from build123d import *

# Parameters (mm, degrees)
CROQUIS1_R              = 1.5
CROQUIS1_R_2            = 1.499997567
CROQUIS1_R_3            = 1.499999659
SALIENTE_EXTRUIR1_DEPTH = 2


with BuildPart() as part:
    # Croquis1 → Saliente-Extruir1 (new body)
    with BuildSketch(Plane.XY):
        with BuildLine():
            Line((-41.931739537, 35.719555975), (-21.729231, 5.566101))
            ThreePointArc((-21.729231, 5.566101), (-20.036969421, 4.8e-08), (-21.729230683, -5.566101))
            Line((-21.729230683, -5.566101), (-41.931739683, -35.719556))
            ThreePointArc((-41.931739683, -35.719556), (-40.113877545, -46.255199079), (-29.502526011, -44.949972494))
            Line((-29.502526011, -44.949972494), (-23.17774412, -37.243793058))
            ThreePointArc((-23.17774412, -37.243793058), (-17.619189001, -31.253867186), (-11.353005357, -26.008708515))
            ThreePointArc((-11.353005357, -26.008708515), (-8.734615775, -24.660409187), (-5.826392082, -24.195532826))
            Line((-5.826392082, -24.195532826), (-8.2e-08, -24.195532826))
            Line((-8.2e-08, -24.195532826), (5.826391918, -24.195532937))
            ThreePointArc((5.826391918, -24.195532937), (8.734615571, -24.66040906), (11.3530052, -26.008708126))
            ThreePointArc((11.3530052, -26.008708126), (17.61928276, -31.253858591), (23.177925918, -37.243793826))
            Line((23.177925918, -37.243793826), (29.502525918, -44.949971826))
            ThreePointArc((29.502525918, -44.949971826), (40.113877545, -46.255199018), (41.931739905, -35.719555809))
            Line((41.931739905, -35.719555809), (40.742639905, -33.944752809))
            ThreePointArc((40.742639905, -33.944752809), (40.308182186, -27.575684066), (45.596686, -23.999999855))
            Line((45.596686, -23.999999855), (66.596686, -23.999999855))
            ThreePointArc((66.596686, -23.999999855), (68.20025333, -23.53546267), (69.307209533, -22.285714318))
            ThreePointArc((69.307209533, -22.285714318), (70.783151209, -20.619383034), (72.921241131, -20.000000062))
            Line((72.921241131, -20.000000062), (107.612588131, -20.000000062))
            ThreePointArc((107.612588131, -20.000000062), (110.006914278, -19.249811766), (111.54509388, -17.267494009))
            ThreePointArc((111.54509388, -17.267494009), (113.827321023, -8.772459026), (114.473968651, -5.93e-07))
            ThreePointArc((114.473968651, -5.93e-07), (113.827320947, 8.772458604), (111.545093444, 17.267494286))
            ThreePointArc((111.545093444, 17.267494286), (110.006913893, 19.249811756), (107.612588, 20))
            Line((107.612588, 20), (72.921241, 20))
            ThreePointArc((72.921241, 20), (70.783151239, 20.619383073), (69.307209698, 22.285714308))
            ThreePointArc((69.307209698, 22.285714308), (68.200253441, 23.535462771), (66.596686, 24))
            Line((66.596686, 24), (45.596686, 24))
            ThreePointArc((45.596686, 24), (40.308182457, 27.575684295), (40.74263977, 33.944752888))
            Line((40.74263977, 33.944752888), (41.93173977, 35.719555888))
            ThreePointArc((41.93173977, 35.719555888), (40.113879793, 46.255201891), (29.502526087, 44.949972367))
            Line((29.502526087, 44.949972367), (23.177744038, 37.243793232))
            ThreePointArc((23.177744038, 37.243793232), (17.619188919, 31.25386736), (11.353005274, 26.008708689))
            ThreePointArc((11.353005274, 26.008708689), (8.734615693, 24.660409361), (5.826392, 24.195533))
            Line((5.826392, 24.195533), (0, 24.195533))
            Line((0, 24.195533), (-5.826392, 24.195533111))
            ThreePointArc((-5.826392, 24.195533111), (-8.734615653, 24.660409234), (-11.353005282, 26.0087083))
            ThreePointArc((-11.353005282, 26.0087083), (-17.619282842, 31.253858765), (-23.177926, 37.243794))
            Line((-23.177926, 37.243794), (-29.502526, 44.949972))
            ThreePointArc((-29.502526, 44.949972), (-40.113877138, 46.255198613), (-41.931739537, 35.719555975))
        make_face()
        with Locations((59.75, -15.25)):
            Circle(CROQUIS1_R, mode=Mode.SUBTRACT)
        with Locations((-15.25, -15.25)):
            Circle(CROQUIS1_R, mode=Mode.SUBTRACT)
        with Locations((35.493242084, -40.033283689)):
            Circle(CROQUIS1_R, mode=Mode.SUBTRACT)
        with Locations((107.612588, -15.5)):
            Circle(CROQUIS1_R, mode=Mode.SUBTRACT)
        with Locations((-35.493241837, -40.033283897)):
            Circle(CROQUIS1_R, mode=Mode.SUBTRACT)
        with Locations((15.25, 15.25)):
            Circle(CROQUIS1_R, mode=Mode.SUBTRACT)
        with Locations((59.75, 15.25)):
            Circle(CROQUIS1_R, mode=Mode.SUBTRACT)
        with Locations((-25.371621, -27.641642)):
            Circle(CROQUIS1_R, mode=Mode.SUBTRACT)
        with Locations((-25.371621, 27.641642)):
            Circle(CROQUIS1_R, mode=Mode.SUBTRACT)
        with Locations((35.493244203, 40.033286852)):
            Circle(CROQUIS1_R_2, mode=Mode.SUBTRACT)
        with Locations((107.612588, 15.5)):
            Circle(CROQUIS1_R, mode=Mode.SUBTRACT)
        with Locations((-35.493241659, 40.033283492)):
            Circle(CROQUIS1_R_3, mode=Mode.SUBTRACT)
        with Locations((90.249999894, -15.249999839)):
            Circle(CROQUIS1_R, mode=Mode.SUBTRACT)
        with Locations((90.24999988, 15.250000209)):
            Circle(CROQUIS1_R, mode=Mode.SUBTRACT)
        with Locations((-15.25, 15.25)):
            Circle(CROQUIS1_R, mode=Mode.SUBTRACT)
        with Locations((25.371621, -27.641642)):
            Circle(CROQUIS1_R, mode=Mode.SUBTRACT)
        with Locations((15.25, -15.25)):
            Circle(CROQUIS1_R, mode=Mode.SUBTRACT)
        with Locations((25.371621, 27.641642)):
            Circle(CROQUIS1_R, mode=Mode.SUBTRACT)
        with BuildLine():
            Line((98.473924, 4.165983), (66.629579, 4.165983))
            ThreePointArc((66.629579, 4.165983), (63.80116944, 6.88617712), (66.409010926, 9.818500341))
            ThreePointArc((66.409010926, 9.818500341), (75.942438766, 10.701918647), (85.446477477, 11.859468837))
            ThreePointArc((85.446477477, 11.859468837), (86.461547798, 11.633214666), (87.383984261, 11.152933833))
            ThreePointArc((87.383984261, 11.152933833), (90.700963866, 10.270378747), (93.80542655, 11.734471854))
            ThreePointArc((93.80542655, 11.734471854), (96.321235225, 12.908534532), (98.995308731, 12.162178491))
            ThreePointArc((98.995308731, 12.162178491), (100.881174903, 9.908695061), (101.470839807, 7.02998457))
            ThreePointArc((101.470839807, 7.02998457), (100.546603986, 4.997112873), (98.473924, 4.165983))
        make_face(mode=Mode.SUBTRACT)
        with BuildLine():
            Line((66.596686, -22), (45.596686, -22))
            ThreePointArc((45.596686, -22), (44.596686, -21), (45.596686, -20))
            Line((45.596686, -20), (66.596686, -20))
            ThreePointArc((66.596686, -20), (67.596686, -21), (66.596686, -22))
        make_face(mode=Mode.SUBTRACT)
        with BuildLine():
            Line((66.596686, 22), (45.596686, 22))
            ThreePointArc((45.596686, 22), (44.596686, 21), (45.596686, 20))
            Line((45.596686, 20), (66.596686, 20))
            ThreePointArc((66.596686, 20), (67.596686, 21), (66.596686, 22))
        make_face(mode=Mode.SUBTRACT)
        with BuildLine():
            Line((98.473923843, -4.165983), (66.629579, -4.165983))
            ThreePointArc((66.629579, -4.165983), (63.801171492, -6.886177421), (66.409011186, -9.818500536))
            ThreePointArc((66.409011186, -9.818500536), (75.942439193, -10.70191878), (85.446478074, -11.859468919))
            ThreePointArc((85.446478074, -11.859468919), (86.461548299, -11.633214373), (87.383984575, -11.152933205))
            ThreePointArc((87.383984575, -11.152933205), (90.700964079, -10.270378355), (93.805426592, -11.734471456))
            ThreePointArc((93.805426592, -11.734471456), (96.32123511, -12.908534134), (98.995308527, -12.162178296))
            ThreePointArc((98.995308527, -12.162178296), (100.881169052, -9.908693453), (101.470829573, -7.029984658))
            ThreePointArc((101.470829573, -7.029984658), (100.546597424, -4.997116386), (98.473923843, -4.165983))
        make_face(mode=Mode.SUBTRACT)
    extrude(amount=SALIENTE_EXTRUIR1_DEPTH)


solid = part.part
Model file for the job. Use its own axes, mm. A direction names the side the tool comes from. Give positions to 0.01 mm unless a question says otherwise; leave off trailing zeros. Loops run counter-clockwise (first coordinate to the right, second up) from the corner with the lowest first, then second, coordinate; pieces in that order, holes last. Notation, with made-up numbers: (50.5, 33.5) -> (77.5, 33.5) arc R24 ccw to (77.5, 66.5) -> close; hole circle Ø10 at (39, 81). An arc over 180 degrees is marked (long way). Use a Markdown table: item, result. Add a question column.
(1) Mould opens along Y. For faces 4 (the flat face through (26.296, -41.043, 0.986)), 5 (the flat face through (17, 1, 2)), 6 (the flat face through (26.384, 41.151, 0.986)), 7 (the cylindrical face through (-34.69, 41.3, 0.99)) say: +Y half, -Y half, draft (parallel to the pull), parting line (faces both ways), or undercut.
(2) Tool access for faces 1 (the flat face through (-26.296, 41.043, 0.986)), 2 (the cylindrical face through (-17.7, -31.33, 0.99)), 3 (the flat face through (-31.97, 20.85, 0.99)): list every direction of +Z, -Z, +X, -X, +Y, -Y with a clear straight run to the whole face (end or side of a thin tool).
(3) Slice it at A-A on x = 59.75. List the corners of the cut face in (y, z), and give its area (3 significant figures).
(4) Slice it at B-B on x = 90.25. List the corners of the cut face in (y, z).
(5) Wall check: line 1 along Y through (x, z) = (68.5, 1.15); line 2 along Y through (x, z) = (93.5, 1.75); line 3 along Y through (x, z) = (-24, 1.3). Give the ranges that are in metal, low to high.
(6) Drop flat-ended pins along their axis: pin 1 Ø1.8 at (x, y) = (-35.49, -40.03) entering from +Z; pin 2 Ø3.5 at (x, y) = (90.25, -15.25) entering from +Z; pin 3 Ø0.6 at (x, z) = (80.5, 1) entering from -Y; pin 4 Ø1 at (x, z) = (2, 0.5) entering from -Y. Give the stop position or say it passes through.
(7) Slice it at C-C on z = 0.6. Give the number of separate pieces and of enclosed holes in the cut face, and give its area (3 significant figures).
Filled sheet:
| question | item | result |
|---|---|---|
| 1 | face 4 | -Y half |
| 1 | face 5 | draft |
| 1 | face 6 | +Y half |
| 1 | face 7 | undercut |
| 2 | face 1 | +Z, -Z, +Y |
| 2 | face 2 | +Z, -Z, -Y |
| 2 | face 3 | +Z, -Z, -X |
| 3 | outline | (-24, 0) -> (-22, 0) -> (-22, 2) -> (-24, 2) -> close; (-20, 0) -> (-16.75, 0) -> (-16.75, 2) -> (-20, 2) -> close; (-13.75, 0) -> (13.75, 0) -> (13.75, 2) -> (-13.75, 2) -> close; (16.75, 0) -> (20, 0) -> (20, 2) -> (16.75, 2) -> close; (22, 0) -> (24, 0) -> (24, 2) -> (22, 2) -> close |
| 3 | area | 76.0 mm2 |
| 4 | outline | (-20, 0) -> (-16.75, 0) -> (-16.75, 2) -> (-20, 2) -> close; (-13.75, 0) -> (-10.25, 0) -> (-10.25, 2) -> (-13.75, 2) -> close; (-4.17, 0) -> (4.17, 0) -> (4.17, 2) -> (-4.17, 2) -> close; (10.25, 0) -> (13.75, 0) -> (13.75, 2) -> (10.25, 2) -> close; (16.75, 0) -> (20, 0) -> (20, 2) -> (16.75, 2) -> close |
| 5 | line 1 | -23.32 to -9.99, -4.17 to 4.17, 9.99 to 23.32 |
| 5 | line 2 | -20 to -11.45, -4.17 to 4.17, 11.45 to 20 |
| 5 | line 3 | -38.25 to -28.25, -27.03 to -8.96, 8.96 to 27.03, 28.25 to 38.25 |
| 6 | pin 1 | through |
| 6 | pin 2 | z = 2 |
| 6 | pin 3 | y = -20 |
| 6 | pin 4 | y = -24.2 |
| 7 | separate pieces | 1 |
| 7 | enclosed holes | 22 |
| 7 | area | 7,460 mm2 |
